from build123d import *

# Parameters (mm, degrees)
SKETCH1_R           = 6.75
BOSS_EXTRUDE1_DEPTH = 21
SKETCH2_R           = 4.8
CUT_EXTRUDE1_DEPTH  = 10
CUT_EXTRUDE2_DEPTH  = 9


with BuildPart() as part:
    # Sketch1 → Boss-Extrude1 (new body)
    with BuildSketch(Plane(origin=(0, 0, 0), x_dir=(1, 0, 0), z_dir=(0, 1, 0))):
        Circle(SKETCH1_R)
    extrude(amount=BOSS_EXTRUDE1_DEPTH)

    # Sketch2 → Cut-Extrude1 (cut)
    with BuildSketch(Plane(origin=(0, 21, 0), x_dir=(1, 0, 0), z_dir=(0, 1, 0))):
        Circle(SKETCH2_R)
    extrude(amount=-CUT_EXTRUDE1_DEPTH, mode=Mode.SUBTRACT)

    # Sketch3 → Cut-Extrude2 (cut)
    with BuildSketch(Plane.XZ):
        with BuildLine():
            Line((-1.29747386, -1.098435971), (1.29747386, -1.098435971))
            ThreePointArc((1.29747386, -1.098435971), (0, 1.7), (-1.29747386, -1.098435971))
        make_face()
    extrude(amount=-CUT_EXTRUDE2_DEPTH, mode=Mode.SUBTRACT)


solid = part.part
Verification items for the finished model (mm, model axes). A direction names the side the tool comes from. Give positions to 0.01 mm unless a question says otherwise; leave off trailing zeros. Write each loop counter-clockwise with the first axis right and the second up, starting at its lowest first coordinate (ties: lowest second). Pieces come first, ordered by that corner, then holes.
(1) Cross-section at A-A (x = 0). Enter the section's corners in (y, z).
(2) Gauge pin test, flat ends, axial feed: pin 1 (1.5 mm diameter, centred on x = -3.5, y = 11, fed in from +Z); pin 2 (5 mm diameter, centred on x = 1, z = -1.5, fed in from +Y); pin 3 (3 mm diameter, centred on x = 2, y = 9.5, fed in from -Z). Record the tip position at first contact, or that the pin passes through.
(3) Access from +Z, -Z, +X, -X, +Y, -Y to the whole of each face (thin tool, end or side, straight path). Record for faces 1 (the face through (0, 0, -2)), 2 (the face through (0, 4, -1.098)), 3 (the face through (2.58, 16.07, -4.05)).
(4) Material ranges on line 1 (X direction, y = 17.5, z = 0); line 2 (Y direction, x = 2.5, z = 3); line 3 (Z direction, x = 0, y = 2.25), recorded low to high.
(5) Cross-section at C-C (y = 3.25). Enter the section's corners in (x, z).
(6) Mould release check, pull along X, two halves, no side actions. Record for faces 4 (the face through (1, 21, -5)), 5 (the face through (-1.46, 10.35, 6.59)), 6 (the face through (0, 11, 0)): +X half, -X half, draft (parallel to the pull), parting line (faces both ways), or undercut.
(7) Cross-section at D-D (z = 2). Enter the section's corners in (x, y), plus the area to 4 significant figures.
(8) Cross-section at B-B (z = 0). Enter the section's corners in (x, y).
Worked out:
1. outline: (0, -6.75) - (21, -6.75) - (21, -4.8) - (11, -4.8) - (11, 4.8) - (21, 4.8) - (21, 6.75) - (0, 6.75) - (0, 1.7) - (9, 1.7) - (9, -1.1) - (0, -1.1) - close
2. pin 1: stops at z = 6.16
2. pin 2: stops at y = 11
2. pin 3: stops at z = -6.73
3. face 1: +Z, -Z, +X, -X, -Y
3. face 2: -Y
3. face 3: +Y
4. line 1: x = -6.75 to -4.8, 4.8 to 6.75
4. line 2: y = 0 to 11
4. line 3: z = -6.75 to -1.1, 1.7 to 6.75
5. outline: circle Ø13.5 at (0, 0); hole (-1.3, -1.1) - (1.3, -1.1) arc R1.7 ccw (long way) to start
6. face 4: draft
6. face 5: parting line
6. face 6: undercut
7. outline: (-6.45, 0) - (6.45, 0) - (6.45, 21) - (4.36, 21) - (4.36, 11) - (-4.36, 11) - (-4.36, 21) - (-6.45, 21) - close
7. area: 183.5 mm2
8. outline: (-6.75, 0) - (-1.7, 0) - (-1.7, 9) - (1.7, 9) - (1.7, 0) - (6.75, 0) - (6.75, 21) - (4.8, 21) - (4.8, 11) - (-4.8, 11) - (-4.8, 21) - (-6.75, 21) - close
